Check sheet for the modelled part. Datum: model origin and axes. Units: mm. Face numbers are marked on the shaded views. A direction names the side the tool comes from. Round coordinates to 2 decimals unless told otherwise and drop trailing zeros. Loops run counter-clockwise (first coordinate to the right, second up) from the corner with the lowest first, then second, coordinate; pieces in that order, holes last. Notation, with made-up numbers: (1.5, 73) - (25.5, 73) arc R24 cw to (25.5, 108) - close; hole circle Ø3 at (32, -26.5). An arc over 180 degrees is marked (long way). Return JSON: item names as keys, results as strings.
from build123d import *

# Parameters (mm, degrees)
F0_W     = 69.07307
F0_H     = 73.183507
F1_DEPTH = 25.4
F3_DEPTH = 6.35


with BuildPart() as f1:
    # F0 (on Top) → F1 (new body)
    with BuildSketch(Plane.XY):
        with Locations((8.906385, -13.518363)):
            Rectangle(F0_W, F0_H)
    extrude(amount=F1_DEPTH)

    # F2 (on face) → F3 (join)
    with BuildSketch(Plane(origin=(-25.63015, 0, 0), x_dir=(0, -1, 0), z_dir=(-1, 0, 0))):
        with BuildLine():
            Line((-23.07339, 0), (-10.37339, 0))
            ThreePointArc((-10.37339, 0), (-14.093134, 8.980256), (-23.07339, 12.7))
            Line((-23.07339, 12.7), (-23.07339, 0))
        make_face()
        with BuildLine():
            ThreePointArc((-23.07339, 12.7), (-32.053646, -8.980256), (-10.37339, 0))
            Line((-10.37339, 0), (-23.07339, 0))
            Line((-23.07339, 0), (-23.07339, 12.7))
        make_face()
        with BuildLine():
            ThreePointArc((50.110117, 12.7), (41.12986, 8.980256), (37.410117, 0))
            Line((37.410117, 0), (50.110117, 0))
            Line((50.110117, 0), (50.110117, 12.7))
        make_face()
        with BuildLine():
            Line((50.110117, 0), (37.410117, 0))
            ThreePointArc((37.410117, 0), (50.110117, -12.7), (62.810117, 0))
            ThreePointArc((62.810117, 0), (59.090373, 8.980256), (50.110117, 12.7))
            Line((50.110117, 12.7), (50.110117, 0))
        make_face()
    extrude(amount=F3_DEPTH)

    # F4: F1 across plane


with BuildPart() as f1_1:
    add(f1.part)
    add(f1.part.mirror(Plane.YZ))


solid = f1_1.part
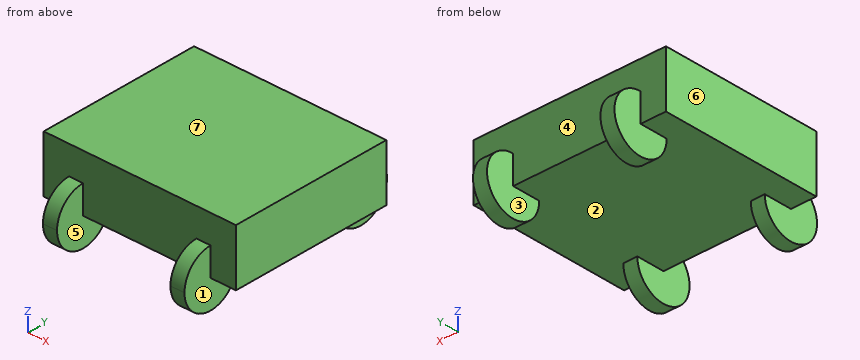
Q1. Sectioned sample at B-B (x = -28). Enter the section's corners in (y, z).
Answer key:
{"outline": "(-50.11, 12.7) arc R12.7 ccw (long way) to (-37.41, 0) - (10.37, 0) arc R12.7 ccw (long way) to (23.07, 12.7) - (23.07, 25.4) - (-50.11, 25.4) - close"}
Q2. Draft check along X on the marked faces 4, 5, 6 and 7. Enter one of: released by +X, released by -X, zero draft, split by the parting line, or undercut.
Answer key:
{"face 4": "undercut", "face 5": "undercut", "face 6": "released by -X", "face 7": "zero draft"}
Q3. Scan lines: probe 1 along X at (y, z) = (-52, -8); probe 2 along Y at (x, z) = (-7.5, 24.5); probe 3 along Y at (x, z) = (31.5, -11). Record each from-to range of solid material in increasing order. Write a range as [from, to].
Answer key:
{"probe 1": "x = [-31.98, -25.63], [25.63, 31.98]", "probe 2": "y = [-50.11, 23.07]", "probe 3": "y = [-56.46, -43.76], [16.73, 29.42]"}
Q4. Tool access check on the marked faces 1, 2 and 3. Record the directions out of +Z, -Z, +X, -X, +Y, -Y that give a thin tool (end or side, any length) a straight path to the whole face; none if there is none.
Answer key:
{"face 1": "-Z, +X, -Y", "face 2": "-Z", "face 3": "-Z, +Y"}
Q5. Depth check by flat-ended pin: P1, Ø22, axis at x = -17, y = -17.5, coming from the -Z side; P2, Ø12.5, axis at x = 1.5, z = 8.5, coming from the +Y side; P3, Ø12.5, axis at x = -9, z = 15.5, coming from the -Y side. Enter the tip coordinate at first touch or a pass-through.
Answer key:
{"P1": "stops at z = 0", "P2": "stops at y = 23.07", "P3": "stops at y = -50.11"}
Q6. Sectioned sample at C-C (y = 13). Enter the section's corners in (x, z), plus the area to 3 significant figures.
Answer key:
{"outline": "(-43.44, 0) - (-31.98, 0) - (-31.98, -7.73) - (-25.63, -7.73) - (-25.63, 0) - (25.63, 0) - (25.63, -7.73) - (31.98, -7.73) - (31.98, 0) - (43.44, 0) - (43.44, 25.4) - (-43.44, 25.4) - close", "area": "2,310 mm²"}
Q7. Sectioned sample at D-D (z = 2). Enter the section's corners in (x, y), plus the area to 3 significant figures.
Answer key:
{"outline": "(-43.44, -50.11) - (-31.98, -50.11) - (-31.98, -62.65) - (-25.63, -62.65) - (-25.63, -50.11) - (25.63, -50.11) - (25.63, -62.65) - (31.98, -62.65) - (31.98, -50.11) - (43.44, -50.11) - (43.44, 23.07) - (31.98, 23.07) - (31.98, 35.61) - (25.63, 35.61) - (25.63, 23.07) - (-25.63, 23.07) - (-25.63, 35.61) - (-31.98, 35.61) - (-31.98, 23.07) - (-43.44, 23.07) - close", "area": "6,680 mm²"}
Q8. Sectioned sample at A-A (y = 29.5). Enter the section's corners in (x, z), plus the area to 3 significant figures.
Answer key:
{"outline": "(-31.98, -10.95) - (-25.63, -10.95) - (-25.63, 10.95) - (-31.98, 10.95) - close; (25.63, -10.95) - (31.98, -10.95) - (31.98, 10.95) - (25.63, 10.95) - close", "area": "278 mm²"}
